Here's how the part is built. I have some questions about the finished solid (model axes, mm). A direction names the side the tool comes from. Coordinates: 2 decimals unless noted, no trailing zeros. Order: outer loops, then holes, each group sorted by start corner. A loop starts at its lowest first (then second) coordinate and runs counter-clockwise, first axis right, second up. Notation, with made-up numbers: (68.25, 85.25) - (77.25, 85.25) arc R12 cw to (77.25, 108.25) - close; hole circle Ø8 at (23.5, -24). An arc over 180 degrees is marked (long way). Answer as CSV lines item,"result". Start each with the question number.
Q1. Thinking about a two-plate mould opening in X: for faces 3 (the face through (-6.87, -0.32, -30.94)), 4 (the face through (-9.4, -25.4, 23.4)), 5 (the face through (-6.3, -22.6, 28.4)), which applies, released by +X, released by -X, zero draft, split by the parting line, or undercut?
Q2. Suppose I cut it at A-A (z = 0). Please give me the cut outline in (x, y), then the cut area to 3 significant figures.
Q3. For pin 1 Ø6 at (y, z) = (-12, -26) entering from +X; pin 2 Ø1 at (x, z) = (-21, 23.5) entering from -Y; pin 3 Ø1 at (x, y) = (-7.5, -14) entering from -Z; pin 4 Ø10 at (x, y) = (-1, -17.5) entering from +Z, each with a flat end and sliding along its axis, tell me the tip position at first contact or that it passes through.
Q4. I need wall thicknesses on line 1 (Z direction, x = 0, y = -13); line 2 (Y direction, x = -1, z = -32.5); line 3 (Z direction, x = 0, y = -23.35). Which ranges of each line are inside material? Lowest first, please.
Q5. Suppose I cut it at D-D (y = -3.5). Please give me the cut outline in (x, z), then the cut area to 3 significant figures.
Q6. Suppose I cut it at B-B (x = 0). Please give me the cut outline in (y, z), then the cut area to 3 significant figures.
Q7. Suppose I cut it at C-C (y = -15.75). Please give me the cut outline in (x, z).
Q8. For faces 1 (the face through (23.704, -1.252, 7.465)), 2 (the face through (32.346, -12.629, 10.186)), which set-ups out of +Z, -Z, +X, -X, +Y, -Y let a thin tool reach every point of the face, with its end or its side?
from build123d import *

# Parameters (mm, degrees)
F0_R     = 36.4522696474
F0_R_2   = 24.8513580129
F1_DEPTH = 25.4
F2_T     = -2.54
F3_SIZE  = 5.08
F4_SIZE  = 5.08


with BuildPart() as f1:
    # F0 (on Front) → F1 (new body)
    with BuildSketch(Plane.XZ):
        Circle(F0_R)
        Circle(F0_R_2, mode=Mode.SUBTRACT)
    extrude(amount=F1_DEPTH)

    # F2
    f2_openings = [f1.faces().sort_by_distance(p)[0] for p in [
        (-24.851358, -12.7, 0),
    ]]
    offset(amount=F2_T, openings=f2_openings)

    # F3
    f3_edges = [f1.edges().sort_by_distance(p)[0] for p in [
        (33.91227, -12.7, 0),
        (-33.91227, -2.54, 0),
        (-33.91227, -22.86, 0),
    ]]
    chamfer(f3_edges, length=F3_SIZE)

    # F4
    f4_edges = [f1.edges().sort_by_distance(p)[0] for p in [
        (36.45227, -12.7, 0),
        (-36.45227, 0, 0),
        (-36.45227, -25.4, 0),
    ]]
    chamfer(f4_edges, length=F4_SIZE)


solid = f1.part
Here are the results:
1,face 3,"split by the parting line"
1,face 4,"zero draft"
1,face 5,"undercut"
2,outline,"(-36.45, -20.32) - (-31.37, -25.4) - (-24.85, -25.4) - (-24.85, -22.86) - (-28.83, -22.86) - (-33.91, -17.78) - (-33.91, -7.62) - (-28.83, -2.54) - (-24.85, -2.54) - (-24.85, 0) - (-31.37, 0) - (-36.45, -5.08) - close; (24.85, -25.4) - (31.37, -25.4) - (36.45, -20.32) - (36.45, -5.08) - (31.37, 0) - (24.85, 0) - (24.85, -2.54) - (28.83, -2.54) - (33.91, -7.62) - (33.91, -17.78) - (28.83, -22.86) - (24.85, -22.86) - close"
2,area,"221 mm²"
3,pin 1,"stops at x = 28.28"
3,pin 2,"stops at y = -25.4"
3,pin 3,"stops at z = -35.77"
3,pin 4,"stops at z = 36.45"
4,line 1,"z = -36.45 to -33.91, 33.91 to 36.45"
4,line 2,"y = -24.26 to -19.18, -6.22 to -1.14"
4,line 3,"z = -33.42 to -24.85, 24.85 to 33.42"
5,outline,"circle Ø69.74 at (0, 0); hole circle Ø59.58 at (0, 0)"
5,area,"1,030 mm²"
6,outline,"(-25.4, -31.37) - (-20.32, -36.45) - (-5.08, -36.45) - (0, -31.37) - (0, -24.85) - (-2.54, -24.85) - (-2.54, -28.83) - (-7.62, -33.91) - (-17.78, -33.91) - (-22.86, -28.83) - (-22.86, -24.85) - (-25.4, -24.85) - close; (-25.4, 24.85) - (-22.86, 24.85) - (-22.86, 28.83) - (-17.78, 33.91) - (-7.62, 33.91) - (-2.54, 28.83) - (-2.54, 24.85) - (0, 24.85) - (0, 31.37) - (-5.08, 36.45) - (-20.32, 36.45) - (-25.4, 31.37) - close"
6,area,"221 mm²"
7,outline,"circle Ø72.9 at (0, 0); hole circle Ø67.82 at (0, 0)"
8,face 1,"+Y, -Y"
8,face 2,"none"
